Can you work these out from the drawing? Everything is in mm from the part's minimum corner. A direction names the side the tool comes from. Round coordinates to 2 decimals unless told otherwise and drop trailing zeros. Loops run counter-clockwise (first coordinate to the right, second up) from the corner with the lowest first, then second, coordinate; pieces in that order, holes last. Notation, with made-up numbers: (81, 31.5) -> (130, 31.5) arc R30 ccw to (130, 58.5) -> close; hole circle Ø3 at (86.25, 81.5). An arc over 180 degrees is marked (long way). One line per item, written item: value.
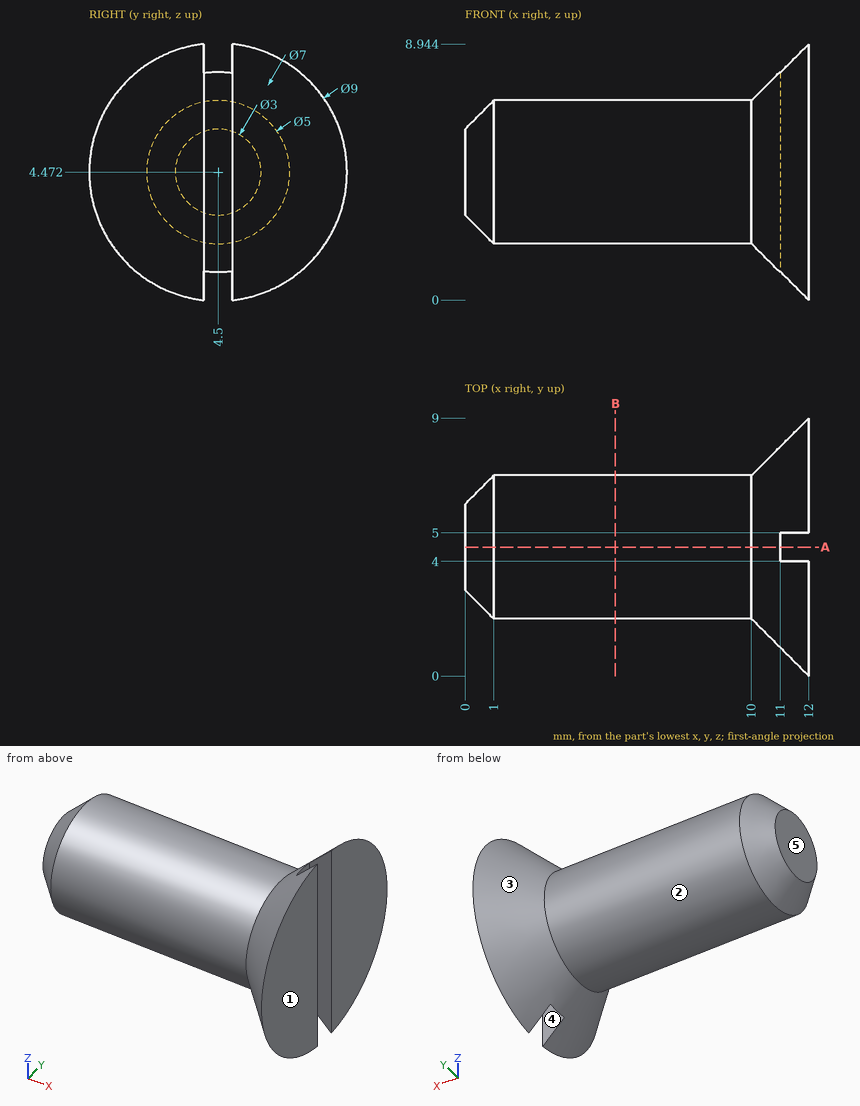
(1) I'm going to push flat-ended pins straight in: pin 1 Ø1 at (y, z) = (1, 5.5) entering from -X; pin 2 Ø0.5 at (x, z) = (11.5, 6.5) entering from -Y (1 decimal); pin 3 Ø0.8 at (x, z) = (11.5, 3.5) entering from +Y. Where does each tip first touch, or does it pass through?
Recorded:
pin 1: x = 10.65
pin 2: y = 0.7
pin 3: y = 8.8
(2) If I drill on L1, parallel to Z at x = 6.25, y = 2.5; L2, parallel to X at y = 1.5, z = 4; L3, parallel to Z at x = 8.75, y = 3, over which ranges is the centre line in solid material (lowest first)?
Recorded:
L1: 2.97 to 5.97
L2: 10.54 to 12
L3: 2.47 to 6.47
(3) Thinking about a two-plate mould opening in Y: for the marked faces 3, 4 and 5, which applies, released by +Y, released by -Y, zero draft, split by the parting line, or undercut?
Recorded:
face 3: split by the parting line
face 4: undercut
face 5: zero draft
(4) For the marked faces 1 and 2, which set-ups out of +Z, -Z, +X, -X, +Y, -Y let a thin tool reach every point of the face, with its end or its side?
Recorded:
face 1: +Z, -Z, +X, +Y, -Y
face 2: -X
(5) If we section it at B-B, the plane x = 5.25: Please give me the cut outline in (y, z), then the cut area to 3 significant figures.
Recorded:
outline: circle Ø5 at (4.5, 4.47)
area: 19.6 mm²
(6) If we section it at A-A, the plane y = 4.5: Please give me the cut outline in (x, z), then the cut area to 3 significant figures.
Recorded:
outline: (0, 2.97) -> (1, 1.97) -> (10, 1.97) -> (11, 0.97) -> (11, 7.97) -> (10, 6.97) -> (1, 6.97) -> (0, 5.97) -> close
area: 55.0 mm²
